Read the model definition and answer for the solid it produces. Units are mm, in the model's axes. Give positions to 0.01 mm unless a question says otherwise; leave off trailing zeros. Order: outer loops, then holes, each group sorted by start corner. A loop starts at its lowest first (then second) coordinate and runs counter-clockwise, first axis right, second up. Notation, with made-up numbers: (31, -23.5) -> (77, -23.5) arc R17 ccw to (77, -7.5) -> close; hole circle Ø7 at (-19.5, 78). An arc over 180 degrees is marked (long way). Use one line per item in the form item = value.
```python
from build123d import *

# Parameters (mm, degrees)
SKETCH1_R           = 1.5
BOSS_EXTRUDE1_DEPTH = 1.3
SKETCH2_R           = 28.5
SKETCH2_R_2         = 1.5
SKETCH2_W           = 90
SKETCH2_H           = 19
CUT_EXTRUDE1_DEPTH  = 10


with BuildPart() as part:
    # Sketch1 → Boss-Extrude1 (new body)
    with BuildSketch(Plane(origin=(0, 0, 0), x_dir=(1, 0, 0), z_dir=(0, 1, 0))):
        with BuildLine():
            Line((-56, -42), (56, -42))
            ThreePointArc((56, -42), (58.828427125, -40.828427125), (60, -38))
            Line((60, -38), (60, 38))
            ThreePointArc((60, 38), (58.828427125, 40.828427125), (56, 42))
            Line((56, 42), (-56, 42))
            ThreePointArc((-56, 42), (-58.828427125, 40.828427125), (-60, 38))
            Line((-60, 38), (-60, -38))
            ThreePointArc((-60, -38), (-58.828427125, -40.828427125), (-56, -42))
        make_face()
        with Locations((-56, 38)):
            Circle(SKETCH1_R, mode=Mode.SUBTRACT)
        with Locations((56, 38)):
            Circle(SKETCH1_R, mode=Mode.SUBTRACT)
        with Locations((56, -38)):
            Circle(SKETCH1_R, mode=Mode.SUBTRACT)
        with Locations((-56, -38)):
            Circle(SKETCH1_R, mode=Mode.SUBTRACT)
    extrude(amount=BOSS_EXTRUDE1_DEPTH)

    # Sketch2 → Cut-Extrude1 (cut)
    with BuildSketch(Plane(origin=(0, 1.3, 0), x_dir=(1, 0, 0), z_dir=(0, 1, 0))):
        with Locations((0, 9.2)):
            Circle(SKETCH2_R)
        with Locations((-25, 34.2)):
            Circle(SKETCH2_R_2)
        with Locations((25, 34.2)):
            Circle(SKETCH2_R_2)
        with Locations((25, -15.8)):
            Circle(SKETCH2_R_2)
        with Locations((-25, -15.8)):
            Circle(SKETCH2_R_2)
        with Locations((0, -32.5)):
            Rectangle(SKETCH2_W, SKETCH2_H)
    extrude(amount=-CUT_EXTRUDE1_DEPTH, mode=Mode.SUBTRACT)


solid = part.part
```
Item 1: The part is cut by section A-A on x = 0. Give the vertices of the cut face in (y, z), and give its area (3 significant figures).
Checks:
outline = (0, -42) -> (1.3, -42) -> (1.3, -37.7) -> (0, -37.7) -> close; (0, 19.3) -> (1.3, 19.3) -> (1.3, 23) -> (0, 23) -> close
area = 10.4 mm²
Item 2: Determine the mould class of faces 1 (the flat face through (-28, 0, -1)), 2 (the cylindrical face through (-55.31, 0.64, 39.33)), 3 (the cylindrical face through (58.859, 0.641, -40.797)) for opening direction Z: +Z half, -Z half, draft (parallel to the pull), parting line (faces both ways), or undercut.
Checks:
face_1 = draft
face_2 = undercut
face_3 = -Z half
Item 3: Given pin 1 Ø2.5 at (x, z) = (25, 15.8) entering from -Y; pin 2 Ø5 at (x, z) = (56, 38) entering from -Y; pin 3 Ø0.6 at (x, y) = (11.5, 0.5) entering from +Z, each flat-ended and moving along its own axis, determine where each tip first touches the part or whether it passes through.
Checks:
pin_1 = through
pin_2 = 0
pin_3 = 23
Item 4: The part is cut by section C-C on z = -13.5. Give the vertices of the cut face in (x, y).
Checks:
outline = (-60, 0) -> (-28.17, 0) -> (-28.17, 1.3) -> (-60, 1.3) -> close; (28.17, 0) -> (60, 0) -> (60, 1.3) -> (28.17, 1.3) -> close
Item 5: Straight lines are drawn through the part: L1, parallel to X at y = 0.35, z = -38; L2, parallel to Z at x = 56, y = 0.55; L3, parallel to X at y = 0.5, z = -8. For each, find the intervals that lie inside material, in ascending order. Write a range as from..to.
Checks:
L1 = -60..-57.5, -54.5..54.5, 57.5..60
L2 = -42..-39.5, -36.5..36.5, 39.5..42
L3 = -60..-28.47, 28.47..60
Item 6: The part is cut by section B-B on y = 0.9. State how many separate pieces and enclosed holes the cut face has, and give its area (3 significant figures).
Checks:
separate_pieces = 1
enclosed_holes = 9
area = 5,750 mm²
Item 7: The part is cut by section D-D on x = 25. Give the vertices of the cut face in (y, z).
Checks:
outline = (0, -42) -> (1.3, -42) -> (1.3, -35.7) -> (0, -35.7) -> close; (0, -32.7) -> (1.3, -32.7) -> (1.3, -22.88) -> (0, -22.88) -> close; (0, 4.48) -> (1.3, 4.48) -> (1.3, 14.3) -> (0, 14.3) -> close; (0, 17.3) -> (1.3, 17.3) -> (1.3, 23) -> (0, 23) -> close
